Work out the finished part from the listing and answer in its coordinate system (mm). Face numbers are marked on the shaded views. A direction names the side the tool comes from. Round coordinates to 2 decimals unless told otherwise and drop trailing zeros. Write each loop counter-clockwise with the first axis right and the second up, starting at its lowest first coordinate (ties: lowest second). Pieces come first, ordered by that corner, then holes. Notation, with made-up numbers: M -17,55 L 25,55 A19 ccw 25,79 Z; hole C -11,-12 d9. An arc over 180 degrees is marked long. Answer in a Markdown table with one row per item.
```python
from build123d import *

# Parameters (mm, degrees)
F0_W       = 228.6
F0_H       = 50.8
F1_DEPTH   = 63.5
F2_R       = 25.4
F3_DEPTH   = 25.4
F5_W       = 133.35
F5_H       = 127
F6_DEPTH   = 50.8
F8_DEPTH   = 127.001
F9_W       = 114.3
F9_H       = 45.4757122113
F10_DEPTH  = 25.4
F11_DEPTH  = 25.4
F13_DEPTH  = 127.001
F14_W      = 45.1612845063
F14_H      = 43.987744288
F14_W_2    = 41.4102021605
F15_DEPTH  = 127.001
F15_FACE_W = 114.3
F15_FACE_H = 14.0218776853
F18_W      = 115.8576831222
F18_H      = 41.3168929517
F19_DEPTH  = 191.9764496515
F20_W      = 76.2
F20_H      = 20.6366241442
F20_W_2    = 5.92666582
F20_H_2    = 15.1961888187
F21_DEPTH  = 6.35
F22_R      = 19.05
F23_DEPTH  = 6.35
F24_R      = 19.05
F25_DEPTH  = 6.35


with BuildPart() as f1:
    # F0 (on Front) → F1 (new body, symmetric)
    with BuildSketch(Plane.XZ):
        with Locations((1.4754496515, 2.5203571515)):
            Rectangle(F0_W, F0_H)
    extrude(amount=F1_DEPTH, both=True)

    # F2 (on face) → F3 (join)
    with BuildSketch(Plane.XZ.offset(63.5)):
        with BuildLine():
            ThreePointArc((-77.8995503485, -22.8796428485), (-52.4995503485, -48.2796428485), (-27.0995503485, -22.8796428485))
            ThreePointArc((-27.0995503485, -22.8796428485), (-52.4995503485, 2.5203571515), (-77.8995503485, -22.8796428485))
        make_face()
        with Locations((52.4995503485, -22.8796428485)):
            Circle(F2_R)
    extrude(amount=-F3_DEPTH)

    # F4: F1 across plane


with BuildPart() as f1_1:
    add(f1.part)
    add(f1.part.mirror(Plane.XZ))

    # F5 (on face) → F6 (join)
    with BuildSketch(Plane.XY.offset(27.9203571515)):
        with Locations((14.1754496515, 0)):
            Rectangle(F5_W, F5_H)
    extrude(amount=F6_DEPTH)

    # F7 (on face) → F8 (cut, through all)
    with BuildSketch(Plane.XZ.offset(63.5)):
        Polygon((80.8504496515, 78.7203571515), (52.4995503485, 78.7203571515), (80.8504496515, 27.9203571515), align=None)
    extrude(amount=-F8_DEPTH, mode=Mode.SUBTRACT)

    # F9 (on face) → F10 (cut)
    with BuildSketch(Plane(origin=(73.5304715342, 0, 41.0365156332), x_dir=(0, 1, 0), z_dir=(0.8732166409, 0, 0.4873322255))):
        with Locations((0, 14.0673470279)):
            Rectangle(F9_W, F9_H)
    extrude(amount=-F10_DEPTH, mode=Mode.SUBTRACT)

    # F11 (add): a face of the model
    f11_faces = [f1_1.faces().sort_by_distance(p)[0] for p in [
        (-52.4995503485, 0, 53.3203571515),
    ]]
    extrude(f11_faces, amount=F11_DEPTH)

    # F12 (on face) → F13 (cut, through all)
    with BuildSketch(Plane.XZ.offset(63.5)):
        Polygon((-77.8995503485, 78.7203571515), (-77.8995503485, 27.9203571515), (-52.4995503485, 78.7203571515), align=None)
    extrude(amount=-F13_DEPTH, mode=Mode.SUBTRACT)

    # F14 (on face) → F15 (cut, through all)
    with BuildSketch(Plane.XZ.offset(63.5)):
        Polygon((-52.4995503485, 27.9203571515), (-52.4995503485, 63.8672858477), (-70.4730146966, 27.9203571515), align=None)
        with Locations((-22.5806422532, 49.9142292955)):
            Rectangle(F14_W, F14_H)
        with Locations((26.6029974446, 49.9142292955)):
            Rectangle(F14_W_2, F14_H)
        Polygon((73.0387046933, 27.9203571515), (52.4995503485, 63.8672858477), (52.4995503485, 27.9203571515), align=None)
    extrude(amount=-F15_DEPTH, mode=Mode.SUBTRACT)

    # F15_face (on face) → F16 (revolve)
    with BuildSketch(Plane(origin=(61.698255806, 0, 24.5037007223), x_dir=(0, -1, 0), z_dir=(-0.4873322255, 0, 0.8732166409))):
        Rectangle(F15_FACE_W, F15_FACE_H)
    revolve(axis=Axis((55.5761873402, 0, 21.0870442932), (0, -1, 0)))

    # F18 (on offset) → F19 (cut, through all)
    with BuildSketch(Plane.YZ.offset(-76.2)):
        with Locations((7.4506e-06, 53.0304405838)):
            Rectangle(F18_W, F18_H)
    extrude(amount=F19_DEPTH, mode=Mode.SUBTRACT)

    # F20 (on face) → F21 (join)
    with BuildSketch(Plane.YZ.offset(115.7754496515)):
        with Locations((0, 2.0944098942)):
            Rectangle(F20_W, F20_H)
        with Locations((-32.59666709, 2.1173956338)):
            Rectangle(F20_W_2, F20_H_2, mode=Mode.SUBTRACT)
        with Locations((-24.4689150477, 2.0539075275)):
            Rectangle(F20_W_2, F20_H_2, mode=Mode.SUBTRACT)
        with Locations((-16.3411630055, 1.9904194212)):
            Rectangle(F20_W_2, F20_H_2, mode=Mode.SUBTRACT)
        with Locations((-8.2134109632, 1.9269313149)):
            Rectangle(F20_W_2, F20_H_2, mode=Mode.SUBTRACT)
        with Locations((-0.085658921, 1.8634432086)):
            Rectangle(F20_W_2, F20_H_2, mode=Mode.SUBTRACT)
        with Locations((8.0420931213, 1.7999551023)):
            Rectangle(F20_W_2, F20_H_2, mode=Mode.SUBTRACT)
        with Locations((16.1698451635, 1.736466996)):
            Rectangle(F20_W_2, F20_H_2, mode=Mode.SUBTRACT)
        with Locations((24.2975972058, 1.6729788898)):
            Rectangle(F20_W_2, F20_H_2, mode=Mode.SUBTRACT)
        with Locations((32.425349248, 1.6094907835)):
            Rectangle(F20_W_2, F20_H_2, mode=Mode.SUBTRACT)
    extrude(amount=F21_DEPTH)

    # F22 (on face) → F23 (join)
    with BuildSketch(Plane(origin=(0, 63.5, 0), x_dir=(-1, 0, 0), z_dir=(0, 1, 0))):
        with BuildLine():
            ThreePointArc((-77.8995503485, -22.8796428485), (-52.4995503485, -48.2796428485), (-27.0995503485, -22.8796428485))
            ThreePointArc((-27.0995503485, -22.8796428485), (-52.4995503485, 2.5203571515), (-77.8995503485, -22.8796428485))
        make_face()
        with Locations((-52.4995503485, -22.8796428485)):
            Circle(F22_R, mode=Mode.SUBTRACT)
        with BuildLine():
            ThreePointArc((77.8995503485, -22.8796428485), (52.4995503485, 2.5203571515), (27.0995503485, -22.8796428485))
            ThreePointArc((27.0995503485, -22.8796428485), (52.4995503485, -48.2796428485), (77.8995503485, -22.8796428485))
        make_face()
        with Locations((52.4995503485, -22.8796428485)):
            Circle(F22_R, mode=Mode.SUBTRACT)
    extrude(amount=F23_DEPTH)

    # F24 (on face) → F25 (join)
    with BuildSketch(Plane.XZ.offset(63.5)):
        with BuildLine():
            ThreePointArc((-77.8995503485, -22.8796428485), (-52.4995503485, -48.2796428485), (-27.0995503485, -22.8796428485))
            ThreePointArc((-27.0995503485, -22.8796428485), (-52.4995503485, 2.5203571515), (-77.8995503485, -22.8796428485))
        make_face()
        with Locations((-52.4995503485, -22.8796428485)):
            Circle(F24_R, mode=Mode.SUBTRACT)
        with BuildLine():
            ThreePointArc((77.8995503485, -22.8796428485), (52.4995503485, 2.5203571515), (27.0995503485, -22.8796428485))
            ThreePointArc((27.0995503485, -22.8796428485), (52.4995503485, -48.2796428485), (77.8995503485, -22.8796428485))
        make_face()
        with Locations((52.4995503485, -22.8796428485)):
            Circle(F24_R, mode=Mode.SUBTRACT)
    extrude(amount=F25_DEPTH)


solid = f1_1.part
```
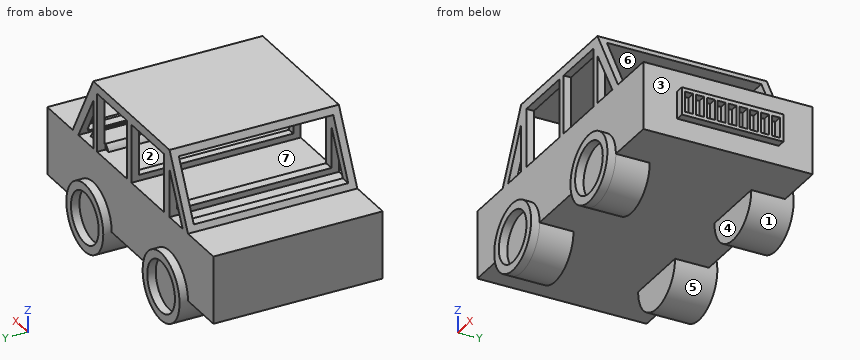
1. The part is cut by section C-C (z = -35). Count the separate pieces of the cut face and the enclosed holes in it, plus the area to 3 significant figures.
Calculated:
| item | result |
|---|---|
| separate pieces | 4 |
| enclosed holes | 0 |
| area | 4,920 mm² |
2. Given pin 1 (1 mm diameter, centred on x = 58, y = -54, fed in from +Z); pin 2 (3 mm diameter, centred on x = 118.5, y = 1, fed in from +Z); pin 3 (8 mm diameter, centred on x = -63, z = 29, fed in from -Y), each flat-ended and moving along its own axis, determine where each tip first touches the part or whether it passes through.
Calculated:
| item | result |
|---|---|
| pin 1 | stops at z = 32.37 |
| pin 2 | stops at z = 12.41 |
| pin 3 | stops at y = -63.5 |
3. Consider line 1 along Z through (x, y) = (-26.5, -28); line 2 along Z through (x, y) = (-5, 60.5); line 3 along Z through (x, y) = (69.5, -3.5). Determine where each line is inside the solid, lowest interval first. Write a range as from..to.
Calculated:
| item | result |
|---|---|
| line 1 | z = -22.88..27.92, 73.69..78.72 |
| line 2 | z = -22.88..27.92, 71.91..78.72 |
| line 3 | z = -22.88..27.92 |
4. The part is cut by section B-B (x = -38.5). Determine the outline of the cut face in (y, z).
Calculated:
| item | result |
|---|---|
| outline | M -69.85,-44.07 L -38.1,-44.07 L -38.1,-22.88 L 38.1,-22.88 L 38.1,-44.07 L 69.85,-44.07 L 69.85,-35.8 L 63.5,-35.8 L 63.5,-9.96 L 69.85,-9.96 L 69.85,-1.69 L 63.5,-1.69 L 63.5,27.92 L -63.5,27.92 L -63.5,-1.69 L -69.85,-1.69 L -69.85,-9.96 L -63.5,-9.96 L -63.5,-35.8 L -69.85,-35.8 Z; M -63.5,71.91 L -57.93,71.91 L -57.93,73.69 L 57.93,73.69 L 57.93,71.91 L 63.5,71.91 L 63.5,78.72 L -63.5,78.72 Z |
5. A tool of negligible diameter and unlimited length cuts with its end or side. For the marked faces 4, 5, 6 and 7, from which of +Z, -Z, +X, -X, +Y, -Y can it reach the whole face along a straight path? Write none if from no direction.
Calculated:
| item | result |
|---|---|
| face 4 | -Z, +X, -X |
| face 5 | +Y |
| face 6 | +X, -X |
| face 7 | +Y, -Y |
6. Determine the mould class of the marked faces 1, 2 and 3 for opening direction Z: released by +Z, released by -Z, zero draft, split by the parting line, or undercut.
Calculated:
| item | result |
|---|---|
| face 1 | split by the parting line |
| face 2 | undercut |
| face 3 | zero draft |
